Geometry: final body of the model. Coordinates: model frame, mm. Face numbers are marked on the shaded views. A direction names the side the tool comes from. Coordinates: 2 decimals unless noted, no trailing zeros. Loops run counter-clockwise (first coordinate to the right, second up) from the corner with the lowest first, then second, coordinate; pieces in that order, holes last. Notation, with made-up numbers: (2.5, -13) - (59.5, -13) arc R26 cw to (59.5, 26) - close; hole circle Ø4 at (82, -6). An arc over 180 degrees is marked (long way). Answer in a Markdown table with one row per item.
from build123d import *

# Parameters (mm, degrees)
CUT_EXTRUDE1_DEPTH = 2


with BuildPart() as part:
    # Sketch1 → Revolve1 (revolve)
    with BuildSketch(Plane(origin=(0, 0, 0), x_dir=(1, 0, 0), z_dir=(0, 1, 0))):
        Polygon((0, 0), (0, 4), (0.2, 4), (2, 2.5), (6.627677822, 2.5), (8, 2), (40, 2), (40, 0), align=None)
    revolve(axis=Axis((40, 0, 0), (-1, 0, 0)))

    # Sketch2 → Cut-Extrude1 (cut)
    with BuildSketch(Plane.ZY):
        Polygon((1.987284991, 1.176448765), (-0.025192021, 2.30926367), (-2.012477012, 1.132814905), (-1.987284991, -1.176448765), (0.025192021, -2.30926367), (2.012477012, -1.132814905), align=None)
    extrude(amount=-CUT_EXTRUDE1_DEPTH, mode=Mode.SUBTRACT)


solid = part.part
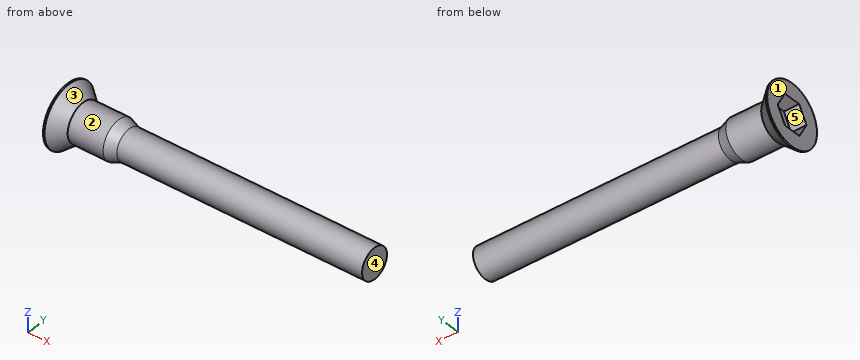
(1) Cut plane A-A on y = 0. Output: boundary loops of the cut face in (x, z).
Verdict:
| item | result |
|---|---|
| outline | (0, -4) - (0.2, -4) - (2, -2.5) - (6.63, -2.5) - (8, -2) - (40, -2) - (40, 2) - (8, 2) - (6.63, 2.5) - (2, 2.5) - (0.2, 4) - (0, 4) - (0, 2) - (2, 2) - (2, -2) - (0, -2) - close |
(2) Pull-direction query (Y, two-part tool) for the marked faces 3, 4 and 5; classes: pulls with the +Y half, pulls with the -Y half, needs draft (parallel to the pull), parting line crosses it, or undercut.
Verdict:
| item | result |
|---|---|
| face 3 | parting line crosses it |
| face 4 | needs draft |
| face 5 | undercut |
(3) Ray query, probe 1 along X at (y, z) = (0, 0.5); probe 2 along Y at (x, z) = (27, 0); probe 3 along Y at (x, z) = (7, -0.5). Return the intervals inside material, ascending.
Verdict:
| item | result |
|---|---|
| probe 1 | x = 2 to 40 |
| probe 2 | y = -2 to 2 |
| probe 3 | y = -2.31 to 2.31 |
(4) Access query for the marked faces 1 and 2. Directions: +Z, -Z, +X, -X, +Y, -Y. A direction counts if a zero-diameter tool reaches every point of the face in a straight line with its end or side. Return the directions, or none.
Verdict:
| item | result |
|---|---|
| face 1 | +Z, -Z, -X, +Y, -Y |
| face 2 | +X |
(5) First-contact query: pin 1 Ø1.5 at (x, z) = (7, 1) entering from -Y; pin 2 Ø4 at (x, z) = (20, -1.5) entering from +Y; pin 3 Ø3 at (x, z) = (11.5, 1) entering from -Y. Flat tips, straight axial feed; report the tip coordinate or a pass-through.
Verdict:
| item | result |
|---|---|
| pin 1 | stops at y = -2.48 |
| pin 2 | stops at y = 2 |
| pin 3 | stops at y = -2 |
(6) Cut plane B-B on x = 37.5. Output: boundary loops of the cut face in (y, z).
Verdict:
| item | result |
|---|---|
| outline | circle Ø4 at (0, 0) |
